Geometry check sheet. Reference: the model listing, model coordinates, mm. A direction names the side the tool comes from. Round coordinates to 2 decimals unless told otherwise and drop trailing zeros. Write each loop counter-clockwise with the first axis right and the second up, starting at its lowest first coordinate (ties: lowest second). Pieces come first, ordered by that corner, then holes.
from build123d import *

# Parameters (mm, degrees)
F0_W     = 19
F0_H     = 19
F0_W_2   = 13.5
F0_H_2   = 13.5
F1_DEPTH = 12.5
F2_W     = 25
F2_H     = 34
F3_DEPTH = 2.5
F4_W     = 25
F4_H     = 2
F5_DEPTH = 30
F6_W     = 2
F6_H     = 25
F7_DEPTH = 20
F8_W     = 32.5
F8_H     = 10
F9_DEPTH = 2


with BuildPart() as f1:
    # F0 (on Front) → F1 (new body, symmetric)
    with BuildSketch(Plane.XZ):
        Rectangle(F0_W, F0_H)
        Rectangle(F0_W_2, F0_H_2, mode=Mode.SUBTRACT)
    extrude(amount=F1_DEPTH, both=True)

    # F2 (on face) → F3 (join)
    with BuildSketch(Plane(origin=(-9.5, 0, 0), x_dir=(0, -1, 0), z_dir=(-1, 0, 0))):
        with Locations((0, -7.5)):
            Rectangle(F2_W, F2_H)
    extrude(amount=-F3_DEPTH)

    # F4 (on face) → F5 (join)
    with BuildSketch(Plane(origin=(-9.5, 0, 0), x_dir=(0, -1, 0), z_dir=(-1, 0, 0))):
        with Locations((0, -23.5)):
            Rectangle(F4_W, F4_H)
    extrude(amount=F5_DEPTH)

    # F6 (on face) → F7 (join)
    with BuildSketch(Plane.XY.offset(-22.5)):
        with Locations((-38.5, 0)):
            Rectangle(F6_W, F6_H)
    extrude(amount=F7_DEPTH)

    # F8 (on face) → F9 (join)
    with BuildSketch(Plane.XZ.offset(12.5)):
        with Locations((-23.25, -19.5)):
            Rectangle(F8_W, F8_H)
    extrude(amount=-F9_DEPTH)


solid = f1.part
1. Release check for a two-part mould opening along X. For faces 6 (the face through (-19, -12.5, -15)), 7 (the face through (-39.5, 0, -14)), 8 (the face through (0, 0, -6.75)) record: +X half, -X half, draft (parallel to the pull), parting line (faces both ways), or undercut.
2. Section check D-D (z = -16.5). Record the cut outline in (x, y).
3. Section check A-A (x = 0). Record the cut outline in (y, z), plus the area to 4 significant figures.
4. Section check B-B (z = -13). Record the cut outline in (x, y).
5. Access from +Z, -Z, +X, -X, +Y, -Y to the whole of each face (thin tool, end or side, straight path). Record for faces 1 (the face through (-7, 0, -17)), 2 (the face through (-24, -10.5, -18)), 3 (the face through (-24, -12, -14.5)), 4 (the face through (-6.75, 0, 0)), 5 (the face through (-39, 0, -2.5)).
6. Depth check by flat-ended pin: pin 1 Ø2 at (x, y) = (-39, -4) entering from +Z; pin 2 Ø4 at (x, z) = (-25.5, -18) entering from +Y; pin 3 Ø1.5 at (y, z) = (8.5, -18) entering from +X. Enter the tip coordinate at first touch or a pass-through.
7. Scan lines: line 1 along X through (y, z) = (-4.25, -1); line 2 along X through (y, z) = (-3.75, -4). Record each from-to range of solid material in increasing order.
8. Section check C-C (y = -9.75). Record the cut outline in (x, z).
Results below:
1. face 6: draft
1. face 7: -X half
1. face 8: undercut
2. outline: (-39.5, -12.5) - (-7, -12.5) - (-7, 12.5) - (-9.5, 12.5) - (-9.5, -10.5) - (-37.5, -10.5) - (-37.5, 12.5) - (-39.5, 12.5) - close
3. outline: (-12.5, -9.5) - (12.5, -9.5) - (12.5, -6.75) - (-12.5, -6.75) - close; (-12.5, 6.75) - (12.5, 6.75) - (12.5, 9.5) - (-12.5, 9.5) - close
3. area: 137.5 mm2
4. outline: (-39.5, -12.5) - (-37.5, -12.5) - (-37.5, 12.5) - (-39.5, 12.5) - close; (-9.5, -12.5) - (-7, -12.5) - (-7, 12.5) - (-9.5, 12.5) - close
5. face 1: -Z, +X, +Y, -Y
5. face 2: +Z, +Y
5. face 3: +Z, +Y, -Y
5. face 4: +Y, -Y
5. face 5: +Z, -X, +Y, -Y
6. pin 1: stops at z = -2.5
6. pin 2: stops at y = -10.5
6. pin 3: stops at x = -7
7. line 1: x = -9.5 to -6.75, 6.75 to 9.5
7. line 2: x = -39.5 to -37.5, -9.5 to -6.75, 6.75 to 9.5
8. outline: (-39.5, -24.5) - (-7, -24.5) - (-7, -9.5) - (9.5, -9.5) - (9.5, 9.5) - (-9.5, 9.5) - (-9.5, -22.5) - (-37.5, -22.5) - (-37.5, -2.5) - (-39.5, -2.5) - close; hole (-6.75, -6.75) - (6.75, -6.75) - (6.75, 6.75) - (-6.75, 6.75) - close
